Drawing for the job (mm, zero at the part's lowest x, y, z). A direction names the side the tool comes from. Give positions to 0.01 mm unless a question says otherwise; leave off trailing zeros. Order: outer loops, then holes, each group sorted by start corner. A loop starts at its lowest first (then second) coordinate and runs counter-clockwise, first axis right, second up. Notation, with made-up numbers: (61, -18) - (115, -18) arc R31 cw to (115, 20) - close; hole circle Ø5 at (64, -15). An arc over 180 degrees is marked (long way). Use CSV: the item, a comma, the result in double quotes. Start each with the question number.
(1) Drop flat-ended pins along their axis: pin 1 Ø2 at (x, y) = (7, 31) entering from -Z; pin 2 Ø6 at (x, z) = (12, 3.5) entering from -Y. Give the stop position or say it passes through.
(2) Probe L1, parallel to Y at x = 14.25, z = 14.5; L2, parallel to Z at x = 4.75, y = 16; L3, parallel to X at y = 47, z = 10 (1 decimal). List the from-to ranges inside material, lowest first.
(3) Band-saw the part on B-B, the plane x = 13.5. Give the cut face in (y, z), then the cut area to 3 significant figures.
(4) Pull direction X, two halves, no side cores. Call the marked faces 3, 4 and 5: +X half, -X half, draft (parallel to the pull), parting line (faces both ways), or undercut.
(5) Band-saw the part on D-D, the plane z = 18.5. Give the cut face in (x, y).
(6) Tool access for the marked faces 1 and 2: list every direction of +Z, -Z, +X, -X, +Y, -Y with a clear straight run to the whole face (end or side of a thin tool).
(7) Band-saw the part on C-C, the plane y = 35.5. Give the cut face in (x, z) (1 decimal).
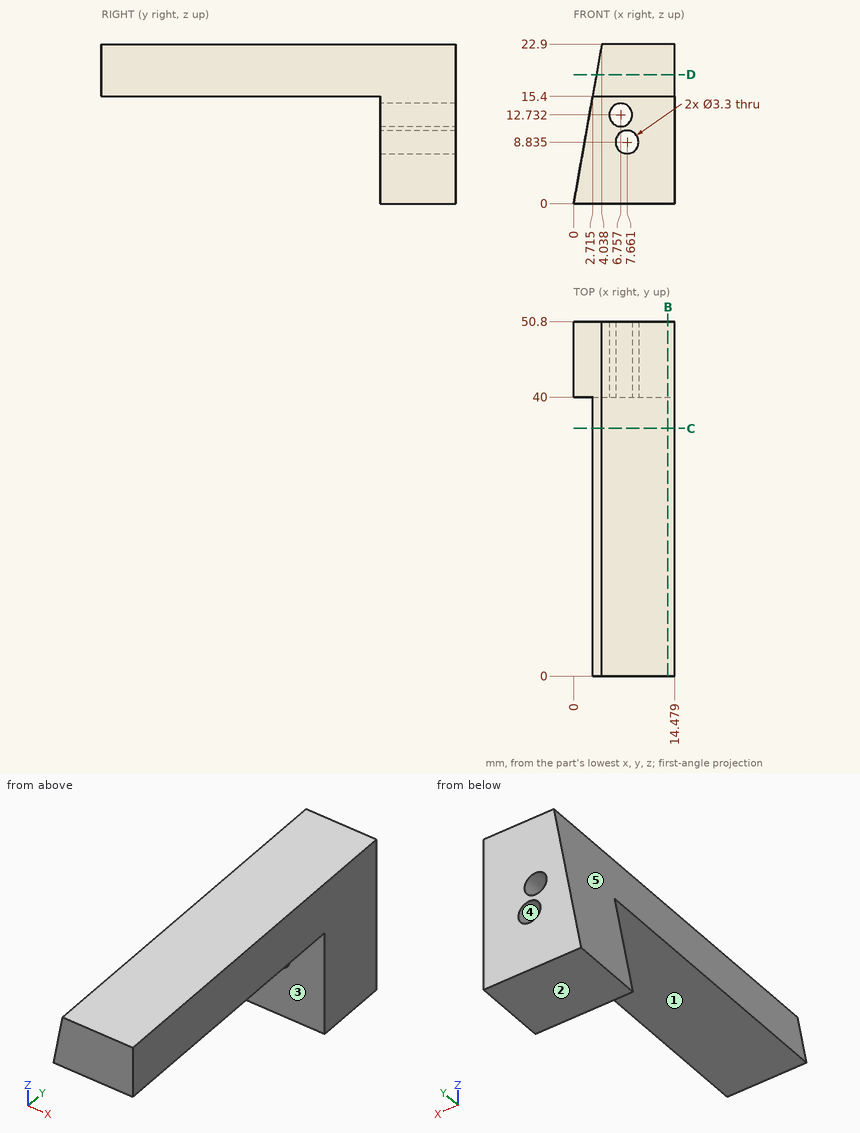
Answer block:
1,pin 1,"stops at z = 15.4"
1,pin 2,"stops at y = 40"
2,L1,"y = 40 to 50.8"
2,L2,"z = 15.4 to 22.9"
2,L3,"x = 1.8 to 6.5, 8.8 to 14.5"
3,outline,"(0, 15.4) - (40, 15.4) - (40, 0) - (50.8, 0) - (50.8, 22.9) - (0, 22.9) - close"
3,area,"547 mm2"
4,face 3,"draft"
4,face 4,"undercut"
4,face 5,"-X half"
5,outline,"(3.26, 0) - (14.48, 0) - (14.48, 50.8) - (3.26, 50.8) - close"
6,face 1,"-Z, +X, -X, -Y"
6,face 2,"-Z, +X, -X, +Y, -Y"
7,outline,"(2.7, 15.4) - (14.5, 15.4) - (14.5, 22.9) - (4, 22.9) - close"
